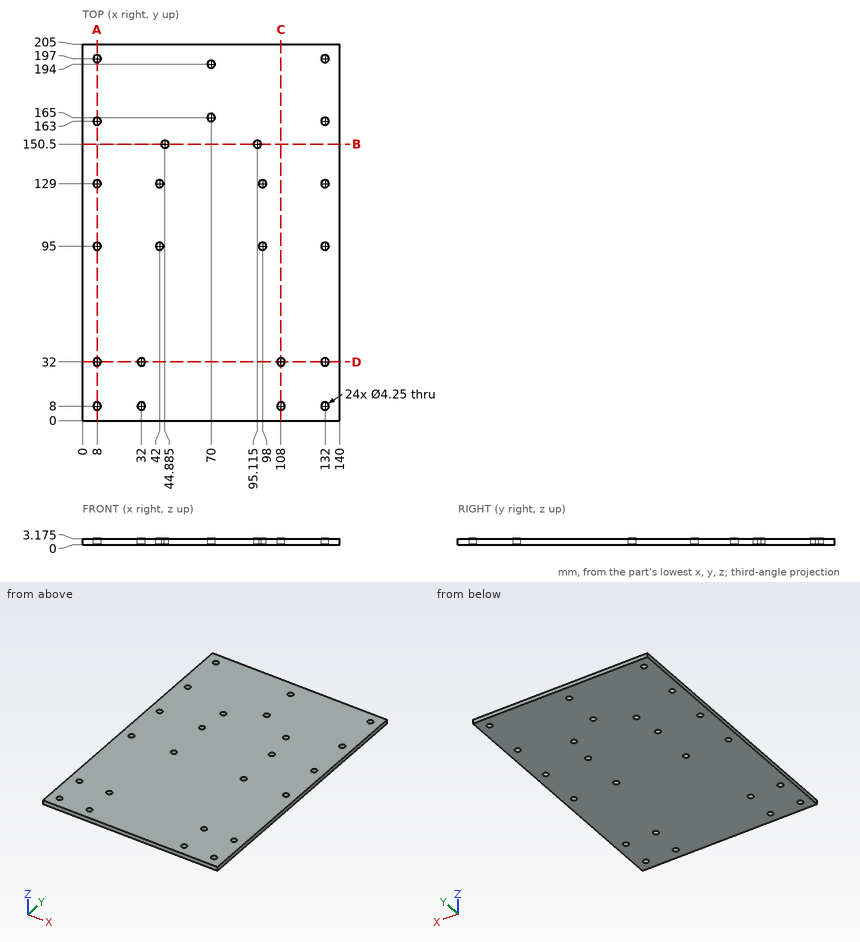
Geometry: see drawing. Coordinates: mm, zero at the bounding-box minimum. Coordinates: 2 decimals unless noted, no trailing zeros. Loops run counter-clockwise (first coordinate to the right, second up) from the corner with the lowest first, then second, coordinate; pieces in that order, holes last.
(1) Section B-B on y = 150.5. Return the cut outline in (x, z) (1 decimal).
(2) First-contact query: pin 1 Ø7 at (x, y) = (42, 95) entering from +Z (3 decimals); pin 2 Ø3.5 at (x, y) = (70, 194) entering from +Z. Flat tips, straight axial feed; report the tip coordinate or a pass-through.
(3) Section D-D on y = 32. Return the cut outline in (x, z) (1 decimal).
(4) Section A-A on x = 8. Return the cut outline in (y, z) (1 decimal), then the cut area to 3 significant figures.
(5) Section C-C on x = 108. Return the cut outline in (y, z) (1 decimal).
(6) Material intervals for probe 1 along X at (y, z) = (197, 0.85) (1 decimal); probe 2 along Y at (x, z) = (70, 2.2) (1 decimal); probe 3 along X at (y, z) = (129, 0.85) (1 decimal), sorted ascending.
Data:
1. outline: (0, 0) - (42.8, 0) - (42.8, 3.2) - (0, 3.2) - close; (47, 0) - (93, 0) - (93, 3.2) - (47, 3.2) - close; (97.2, 0) - (140, 0) - (140, 3.2) - (97.2, 3.2) - close
2. pin 1: stops at z = 3.175
2. pin 2: passes through
3. outline: (0, 0) - (5.9, 0) - (5.9, 3.2) - (0, 3.2) - close; (10.1, 0) - (29.9, 0) - (29.9, 3.2) - (10.1, 3.2) - close; (34.1, 0) - (105.9, 0) - (105.9, 3.2) - (34.1, 3.2) - close; (110.1, 0) - (129.9, 0) - (129.9, 3.2) - (110.1, 3.2) - close; (134.1, 0) - (140, 0) - (140, 3.2) - (134.1, 3.2) - close
4. outline: (0, 0) - (5.9, 0) - (5.9, 3.2) - (0, 3.2) - close; (10.1, 0) - (29.9, 0) - (29.9, 3.2) - (10.1, 3.2) - close; (34.1, 0) - (92.9, 0) - (92.9, 3.2) - (34.1, 3.2) - close; (97.1, 0) - (126.9, 0) - (126.9, 3.2) - (97.1, 3.2) - close; (131.1, 0) - (160.9, 0) - (160.9, 3.2) - (131.1, 3.2) - close; (165.1, 0) - (194.9, 0) - (194.9, 3.2) - (165.1, 3.2) - close; (199.1, 0) - (205, 0) - (205, 3.2) - (199.1, 3.2) - close
4. area: 570 mm2
5. outline: (0, 0) - (5.9, 0) - (5.9, 3.2) - (0, 3.2) - close; (10.1, 0) - (29.9, 0) - (29.9, 3.2) - (10.1, 3.2) - close; (34.1, 0) - (205, 0) - (205, 3.2) - (34.1, 3.2) - close
6. probe 1: x = 0 to 5.9, 10.1 to 129.9, 134.1 to 140
6. probe 2: y = 0 to 162.9, 167.1 to 191.9, 196.1 to 205
6. probe 3: x = 0 to 5.9, 10.1 to 39.9, 44.1 to 95.9, 100.1 to 129.9, 134.1 to 140
